Geometry: final body of the model. Coordinates: model frame, mm. Coordinates: 2 decimals unless noted, no trailing zeros. Order: outer loops, then holes, each group sorted by start corner. A loop starts at its lowest first (then second) coordinate and runs counter-clockwise, first axis right, second up. Notation, with made-up numbers: M 42,7 L 66,7 A19 cw 66,29 Z; hole C 7.5,71 d8. An arc over 180 degrees is marked long. Use CSV: the item, a comma, the result in double quotes. Start each with the question number.
Q1. Ray query, probe 1 along X at (y, z) = (479, 1.5); probe 2 along X at (y, z) = (-515.5, -8.5); probe 3 along Z at (x, y) = (6, 283) (3 decimals). Return the intervals inside material, ascending.
Q2. Section query A-A, the plane x = 0. Output: boundary loops of the cut face in (y, z) (3 decimals).
Q3. Section query C-C, the plane z = 6.5. State how many separate pieces and enclosed holes the cut face has, and give its area (3 significant figures).
Q4. First-contact query: P1, Ø2.5, axis at x = -12.5, y = 75, coming from the +Z side; P2, Ø6.5, axis at x = -1, y = -614, coming from the -Z side (3 decimals). Flat tips, straight axial feed; report the tip coordinate or a pass-through.
Q5. Section query B-B, the plane y = -404.5. Output: boundary loops of the cut face in (x, z) (3 decimals), and give its area (3 significant figures).
from build123d import *

# Parameters (mm, degrees)
SKETCH1_W           = 19.05
SKETCH1_H           = 1270
BOSS_EXTRUDE1_DEPTH = 19.05
SKETCH2_R           = 6.35
CUT_EXTRUDE1_DEPTH  = 636.571243056
SKETCH4_W           = 12.7
SKETCH4_H           = 12.7
CUT_EXTRUDE2_DEPTH  = 1271.178581194
SKETCH5_R           = 1.905
CUT_EXTRUDE3_DEPTH  = 636.571243056
SKETCH6_R           = 4.1275
CUT_EXTRUDE4_DEPTH  = 7.747


with BuildPart() as part:
    # Sketch1 → Boss-Extrude1 (new, symmetric)
    with BuildSketch(Plane(origin=(0, 0, 0), x_dir=(0, 0, -1), z_dir=(1, 0, 0))):
        Rectangle(SKETCH1_W, SKETCH1_H)
    extrude(amount=BOSS_EXTRUDE1_DEPTH, both=True)

    # Sketch2 → Cut-Extrude1 (cut, through all)
    with BuildSketch(Plane.XY.offset(9.525)):
        with Locations((0, -574.675)):
            Circle(SKETCH2_R)
    extrude(amount=-CUT_EXTRUDE1_DEPTH, mode=Mode.SUBTRACT)

    # Sketch4 → Cut-Extrude2 (cut, through all)
    with BuildSketch(Plane(origin=(0, 635, 0), x_dir=(1, 0, 0), z_dir=(0, 1, 0))):
        with Locations((0, 9.525)):
            Rectangle(SKETCH4_W, SKETCH4_H)
    extrude(amount=-CUT_EXTRUDE2_DEPTH, mode=Mode.SUBTRACT)

    # Sketch5 → Cut-Extrude3 (cut, through all)
    with BuildSketch(Plane.XY.offset(9.525)):
        with Locations((-11.43, 513.302135886)):
            Circle(SKETCH5_R)
        with Locations((11.43, 478.263647874)):
            Circle(SKETCH5_R)
        with Locations((-11.43, 463.345550332)):
            Circle(SKETCH5_R)
        with Locations((11.43, 430.113859098)):
            Circle(SKETCH5_R)
        with Locations((-11.43, 407.064148942)):
            Circle(SKETCH5_R)
        with Locations((11.43, 379.842698104)):
            Circle(SKETCH5_R)
        with Locations((-11.43, 366.551491472)):
            Circle(SKETCH5_R)
        with Locations((11.43, 316.418969048)):
            Circle(SKETCH5_R)
        with Locations((-11.43, 535.422112699)):
            Circle(SKETCH5_R)
        with Locations((-11.43, 552.28498253)):
            Circle(SKETCH5_R)
        with Locations((-11.43, 562.430692594)):
            Circle(SKETCH5_R)
        with Locations((11.43, 165.149796436)):
            Circle(SKETCH5_R)
        with Locations((11.43, 108.45633512)):
            Circle(SKETCH5_R)
        with Locations((11.43, 79.058526758)):
            Circle(SKETCH5_R)
        with Locations((11.43, 49.653866377)):
            Circle(SKETCH5_R)
        with Locations((11.43, 27.043187605)):
            Circle(SKETCH5_R)
        with Locations((11.43, -2.198894726)):
            Circle(SKETCH5_R)
        with Locations((-11.43, 74.386924519)):
            Circle(SKETCH5_R)
        with Locations((-11.43, 137.013245544)):
            Circle(SKETCH5_R)
        with Locations((-11.43, 212.596714918)):
            Circle(SKETCH5_R)
        with Locations((-11.43, 275.179690854)):
            Circle(SKETCH5_R)
    extrude(amount=-CUT_EXTRUDE3_DEPTH, mode=Mode.SUBTRACT)

    # Sketch6 → Cut-Extrude4 (cut)
    with BuildSketch(Plane.XY.offset(9.525)):
        with Locations((-11.43, 513.302135886)):
            Circle(SKETCH6_R)
        with Locations((11.43, 478.263647874)):
            Circle(SKETCH6_R)
        with Locations((-11.43, 463.345550332)):
            Circle(SKETCH6_R)
        with Locations((11.43, 430.113859098)):
            Circle(SKETCH6_R)
        with Locations((11.43, 379.842698104)):
            Circle(SKETCH6_R)
        with Locations((11.43, 316.418969048)):
            Circle(SKETCH6_R)
        with Locations((-11.43, 366.551491472)):
            Circle(SKETCH6_R)
        with Locations((-11.43, 407.064148942)):
            Circle(SKETCH6_R)
        with Locations((-11.43, 562.430692594)):
            Circle(SKETCH6_R)
        with Locations((-11.43, 552.28498253)):
            Circle(SKETCH6_R)
        with Locations((-11.43, 535.422112699)):
            Circle(SKETCH6_R)
        with Locations((-11.43, 275.179690854)):
            Circle(SKETCH6_R)
        with Locations((-11.43, 212.596714918)):
            Circle(SKETCH6_R)
        with Locations((11.43, 165.149796436)):
            Circle(SKETCH6_R)
        with Locations((-11.43, 137.013245544)):
            Circle(SKETCH6_R)
        with Locations((11.43, 108.45633512)):
            Circle(SKETCH6_R)
        with Locations((11.43, 79.058526758)):
            Circle(SKETCH6_R)
        with Locations((-11.43, 74.386924519)):
            Circle(SKETCH6_R)
        with Locations((11.43, 49.653866377)):
            Circle(SKETCH6_R)
        with Locations((11.43, 27.043187605)):
            Circle(SKETCH6_R)
        with Locations((11.43, -2.198894726)):
            Circle(SKETCH6_R)
    extrude(amount=-CUT_EXTRUDE4_DEPTH, mode=Mode.SUBTRACT)


solid = part.part
Responses:
1,probe 1,"x = -19.05 to 9.67, 13.19 to 19.05"
1,probe 2,"x = -19.05 to -6.35, 6.35 to 19.05"
1,probe 3,"z = -3.175 to 9.525"
2,outline,"M -635,-3.175 L -581.025,-3.175 L -581.025,9.525 L -635,9.525 Z; M -568.325,-3.175 L 635,-3.175 L 635,9.525 L -568.325,9.525 Z"
3,separate pieces,"1"
3,enclosed holes,"22"
3,area,"47,100 mm²"
4,P1,"stops at z = 1.78"
4,P2,"stops at z = -3.175"
5,outline,"M -19.05,-9.525 L -6.35,-9.525 L -6.35,-3.175 L 6.35,-3.175 L 6.35,-9.525 L 19.05,-9.525 L 19.05,9.525 L -19.05,9.525 Z"
5,area,"645 mm²"
